The listing builds one solid part. Answer for the finished solid, in the listing's coordinates (mm). A direction names the side the tool comes from. Round coordinates to 2 decimals unless told otherwise and drop trailing zeros. Write each loop counter-clockwise with the first axis right and the second up, starting at its lowest first coordinate (ties: lowest second). Pieces come first, ordered by that corner, then holes.
(1) A cutting plane is placed at D-D, the plane z = 37. Give the vertices of the cut face in (x, y).
(2) Find the intervals of material crossed by probe 1 along Y at (x, z) = (36.6, 0.8); probe 2 along X at (y, z) = (-31, 4); probe 3 along X at (y, z) = (2, 6), in increasing order.
(3) The mould has two halves that part along X. Classify faces 1 (the face through (-10, 1, 0)), 2 (the face through (38.195, 23, 23)), 3 (the face through (57.377, -1, 3)): +X half, -X half, draft (parallel to the pull), parting line (faces both ways), or undercut.
(4) A cutting plane is placed at B-B, the plane y = 31.5. Give the vertices of the cut face in (x, z), and give its area (3 significant figures).
(5) For faces 4 (the face through (34.3, -17, 7)), 5 (the face through (-50.445, 10.547, 2.535)), 6 (the face through (-3.4, 19, 22)), determine the directions among +Z, -Z, +X, -X, +Y, -Y from which every point of the face is accessible in a straight line to the end or side of a thin tool.
(6) A cutting plane is placed at C-C, the plane z = 8. Give the vertices of the cut face in (x, y).
(7) Each of these flat-tipped pins is pushed along its axis until it touches: pin 1 Ø4 at (x, y) = (-41.5, 7) entering from +Z; pin 2 Ø2.5 at (x, y) = (5.6, -31.5) entering from -Z; pin 3 Ø3.5 at (x, z) = (-1.5, 27) entering from -Y; pin 4 Ø1 at (y, z) = (23, 28) entering from -X. Where does it stop, or does it pass through?
(8) A cutting plane is placed at A-A, the plane x = 36.6. Give the vertices of the cut face in (y, z), and give its area (3 significant figures).
from build123d import *

# Parameters (mm, degrees)
SKETCH_1_W          = 150
SKETCH_1_H          = 84
EXTRUDE_1_DEPTH     = 5
SKETCH_2_W          = 49
SKETCH_2_H          = 49
EXTRUDE_2_DEPTH     = 35
SKETCH_3_W          = 35
SKETCH_3_H          = 30
CUT_EXTRUDE_1_DEPTH = 21
SKETCH_4_W          = 30
SKETCH_4_H          = 35
CUT_EXTRUDE_2_DEPTH = 21
FILLET_1_R          = 0.8
CUT_EXTRUDE_3_DEPTH = 21
SKETCH_6_W          = 27.415053397
SKETCH_6_H          = 84
CUT_EXTRUDE_4_DEPTH = 21
FILLET_2_R          = 0.8
EXTRUDE_5_DEPTH     = 5
SKETCH_12_R         = 1.65
CUT_EXTRUDE_5_DEPTH = 10
SKETCH_13_R         = 3
CUT_EXTRUDE_6_DEPTH = 3


with BuildPart() as part:
    # 草图1 → 凸台-拉伸1 (new body)
    with BuildSketch(Plane.XY):
        Rectangle(SKETCH_1_W, SKETCH_1_H)
    extrude(amount=EXTRUDE_1_DEPTH)

    # 草图2 → 凸台-拉伸2 (add)
    with BuildSketch(Plane.XY.offset(5)):
        with Locations((21.1, 0)):
            Rectangle(SKETCH_2_W, SKETCH_2_H)
        Polygon((0, 0), (0, 21.1), (42.2, 21.1), (42.2, -21.1), (0, -21.1), align=None, mode=Mode.SUBTRACT)
    extrude(amount=EXTRUDE_2_DEPTH)

    # 草图3 → 切除-拉伸1 (cut)
    with BuildSketch(Plane.ZY.offset(3.4)):
        with Locations((22.5, 0.18053777)):
            Rectangle(SKETCH_3_W, SKETCH_3_H)
    extrude(amount=-CUT_EXTRUDE_1_DEPTH, mode=Mode.SUBTRACT)

    # 草图4 → 切除-拉伸2 (cut)
    with BuildSketch(Plane(origin=(0, 24.5, 0), x_dir=(1, 0, 0), z_dir=(0, 1, 0))):
        with Locations((23.194652979, -22.5)):
            Rectangle(SKETCH_4_W, SKETCH_4_H)
    extrude(amount=-CUT_EXTRUDE_2_DEPTH, mode=Mode.SUBTRACT)

    # 圆角1
    fillet_1_edges = [part.edges().sort_by_distance(p)[0] for p in [
        (45.6, -24.5, 22.5),
        (45.6, 24.5, 22.5),
        (-3.4, 24.5, 22.5),
        (-3.4, -24.5, 22.5),
        (75, -42, 2.5),
        (-75, -42, 2.5),
        (-75, 42, 2.5),
        (75, 42, 2.5),
    ]]
    fillet(fillet_1_edges, radius=FILLET_1_R)

    # 草图5 → 切除-拉伸3 (cut)
    with BuildSketch(Plane.XY.offset(5)):
        with BuildLine():
            Line((-48.149197029, 26.428665041), (-64.478381839, 3.358073657))
            ThreePointArc((-64.478381839, 3.358073657), (-66.677650185, 2.98177299), (-67.053950852, 5.181041335))
            Line((-67.053950852, 5.181041335), (-50.724766042, 28.251632719))
            ThreePointArc((-50.724766042, 28.251632719), (-48.525497697, 28.627933386), (-48.149197029, 26.428665041))
        make_face()
        with BuildLine():
            Line((-44.360375577, 23.74696674), (-60.689560387, 0.676375357))
            ThreePointArc((-60.689560387, 0.676375357), (-62.535750423, 0.360487328), (-62.851638452, 2.206677363))
            Line((-62.851638452, 2.206677363), (-46.522453641, 25.277268747))
            ThreePointArc((-46.522453641, 25.277268747), (-44.676263606, 25.593156775), (-44.360375577, 23.74696674))
        make_face()
        with BuildLine():
            Line((-39.434375371, 20.209781933), (-56.396344169, -2.412929875))
            ThreePointArc((-56.396344169, -2.412929875), (-58.505226428, -2.71450716), (-58.806803713, -0.605624901))
            Line((-58.806803713, -0.605624901), (-41.844834915, 22.017086907))
            ThreePointArc((-41.844834915, 22.017086907), (-39.735952656, 22.318664192), (-39.434375371, 20.209781933))
        make_face()
        with BuildLine():
            Line((-34.352361813, 16.39940959), (-51.314330611, -6.223302218))
            ThreePointArc((-51.314330611, -6.223302218), (-53.573704294, -6.546400285), (-53.896802361, -4.287026602))
            Line((-53.896802361, -4.287026602), (-36.934833563, 18.335685206))
            ThreePointArc((-36.934833563, 18.335685206), (-34.67545988, 18.658783273), (-34.352361813, 16.39940959))
        make_face()
        with BuildLine():
            Line((-28.599059516, 12.085720989), (-45.333964099, -10.234148128))
            ThreePointArc((-45.333964099, -10.234148128), (-47.413554704, -10.531536607), (-47.710943184, -8.451946002))
            Line((-47.710943184, -8.451946002), (-30.976038601, 13.867923114))
            ThreePointArc((-30.976038601, 13.867923114), (-28.896447996, 14.165311594), (-28.599059516, 12.085720989))
        make_face()
        with BuildLine():
            Line((-22.701866689, 7.664146707), (-39.300291247, -14.473694703))
            ThreePointArc((-39.300291247, -14.473694703), (-41.643790703, -14.80882304), (-41.97891904, -12.465323584))
            Line((-41.97891904, -12.465323584), (-25.380494482, 9.672517826))
            ThreePointArc((-25.380494482, 9.672517826), (-23.036995026, 10.007646163), (-22.701866689, 7.664146707))
        make_face()
    extrude(amount=-CUT_EXTRUDE_3_DEPTH, mode=Mode.SUBTRACT)

    # 草图6 → 切除-拉伸4 (cut)
    with BuildSketch(Plane.XY.offset(5)):
        with Locations((71.084387087, 0)):
            Rectangle(SKETCH_6_W, SKETCH_6_H)
    extrude(amount=-CUT_EXTRUDE_4_DEPTH, mode=Mode.SUBTRACT)

    # 圆角2
    fillet_2_edges = [part.edges().sort_by_distance(p)[0] for p in [
        (57.376860388, -42, 2.5),
        (57.376860388, 42, 2.5),
    ]]
    fillet(fillet_2_edges, radius=FILLET_2_R)

    # 草图10 → 凸台-拉伸5 (add)
    with BuildSketch(Plane.XY.offset(5)):
        Polygon((0, 21.1), (0, -21.1), (8, -21.1), (8, -13.15), (34.3, -13.15), (34.3, -21.1), (42.2, -21.1), (42.2, 21.1), align=None)
    extrude(amount=EXTRUDE_5_DEPTH)

    # 草图12 → 切除-拉伸5 (cut)
    with BuildSketch(Plane.XY.offset(5)):
        with Locations((5.6, -31.5)):
            Circle(SKETCH_12_R)
        with Locations((5.6, 31.5)):
            Circle(SKETCH_12_R)
        with Locations((36.6, -31.5)):
            Circle(SKETCH_12_R)
        with Locations((36.6, 31.5)):
            Circle(SKETCH_12_R)
    extrude(amount=-CUT_EXTRUDE_5_DEPTH, mode=Mode.SUBTRACT)

    # 草图13 → 切除-拉伸6 (cut)
    with BuildSketch(Plane(origin=(0, 0, 0), x_dir=(-1, 0, 0), z_dir=(0, 0, -1))):
        with Locations((-5.6, 31.5)):
            Circle(SKETCH_13_R)
        with Locations((-5.6, -31.5)):
            Circle(SKETCH_13_R)
        with Locations(Location((-36.6, -31.5, 0), (0, 0, 180))):
            Circle(SKETCH_13_R)
        with Locations(Location((-36.6, 31.5, 0), (0, 0, 180))):
            Circle(SKETCH_13_R)
    extrude(amount=-CUT_EXTRUDE_6_DEPTH, mode=Mode.SUBTRACT)


solid = part.part
Solutions:
1. outline: (-3.4, -23.7) arc R0.8 ccw to (-2.6, -24.5) - (44.8, -24.5) arc R0.8 ccw to (45.6, -23.7) - (45.6, 23.7) arc R0.8 ccw to (44.8, 24.5) - (38.19, 24.5) - (38.19, 21.1) - (42.2, 21.1) - (42.2, -21.1) - (0, -21.1) - (0, -14.82) - (-3.4, -14.82) - close; (-3.4, 15.18) - (0, 15.18) - (0, 21.1) - (8.19, 21.1) - (8.19, 24.5) - (-2.6, 24.5) arc R0.8 ccw to (-3.4, 23.7) - close
2. probe 1: y = -42 to -34.5, -28.5 to 28.5, 34.5 to 42
2. probe 2: x = -75 to 4.03, 7.17 to 35.03, 38.17 to 57.38
2. probe 3: x = 0 to 45.6
3. face 1: draft
3. face 2: undercut
3. face 3: +X half
4. outline: (-75, 0) - (2.6, 0) - (2.6, 3) - (3.95, 3) - (3.95, 5) - (-75, 5) - close; (7.25, 3) - (8.6, 3) - (8.6, 0) - (33.6, 0) - (33.6, 3) - (34.95, 3) - (34.95, 5) - (7.25, 5) - close; (38.25, 3) - (39.6, 3) - (39.6, 0) - (57.38, 0) - (57.38, 5) - (38.25, 5) - close
4. area: 613 mm2
5. face 4: +Z
5. face 5: +Z, -Z
5. face 6: +Z, -X, +Y, -Y
6. outline: (-3.4, -23.7) arc R0.8 ccw to (-2.6, -24.5) - (44.8, -24.5) arc R0.8 ccw to (45.6, -23.7) - (45.6, 23.7) arc R0.8 ccw to (44.8, 24.5) - (38.19, 24.5) - (38.19, 21.1) - (8.19, 21.1) - (8.19, 24.5) - (-2.6, 24.5) arc R0.8 ccw to (-3.4, 23.7) - (-3.4, 15.18) - (0, 15.18) - (0, -14.82) - (-3.4, -14.82) - close; hole (8, -21.1) - (34.3, -21.1) - (34.3, -13.15) - (8, -13.15) - close
7. pin 1: stops at z = 5
7. pin 2: passes through
7. pin 3: stops at y = -24.5
7. pin 4: stops at x = -3.4
8. outline: (-42, 0) - (-34.5, 0) - (-34.5, 3) - (-33.15, 3) - (-33.15, 5) - (-42, 5) - close; (-29.85, 3) - (-28.5, 3) - (-28.5, 0) - (28.5, 0) - (28.5, 3) - (29.85, 3) - (29.85, 5) - (21.1, 5) - (21.1, 10) - (-21.1, 10) - (-21.1, 40) - (-24.5, 40) - (-24.5, 5) - (-29.85, 5) - close; (33.15, 3) - (34.5, 3) - (34.5, 0) - (42, 0) - (42, 5) - (33.15, 5) - close
8. area: 701 mm2
